Design review of the part built by this model. Coordinates are the model's own, in mm. Face numbers are marked on the shaded views. Give positions to 0.01 mm unless a question says otherwise; leave off trailing zeros. Write each loop counter-clockwise with the first axis right and the second up, starting at its lowest first coordinate (ties: lowest second). Pieces come first, ordered by that corner, then holes. Notation, with made-up numbers: (-6.5, 32) -> (5.5, 32) arc R14 ccw to (5.5, 54) -> close; hole circle Ø5 at (-6, 48). An arc over 180 degrees is marked (long way). Return JSON: item names as keys, results as strings. Group by question number.
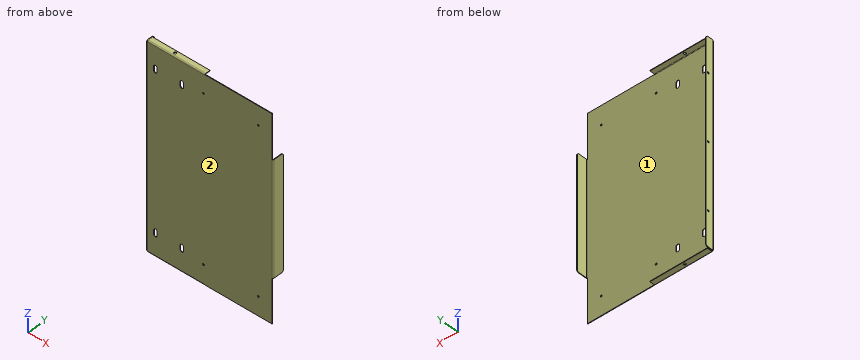
from build123d import *

# Parameters (mm, degrees)
SM_BASE_FLANGE_1_DEPTH   = 381
SKETCH_6_R               = 3.5
CUT_EXTRUDE_1_DEPTH      = 10
SKETCH_7_R               = 3.25
CUT_EXTRUDE_2_DEPTH      = 10
SM_EDGE_FLANGE_2_DEPTH   = 430
OTHER_START              = -2
OTHER_1_DEPTH            = 2
OTHER_START_2            = 477
OTHER_1_2_DEPTH          = 2
SM_START                 = -2
SM_EDGE_FLANGE_4_DEPTH   = 223
SM_EDGE_FLANGE_4_2_DEPTH = 4
SM_START_2               = 220
SM_EDGE_FLANGE_4_3_DEPTH = 1
SM_START_3               = 2
SM_EDGE_FLANGE_4_4_DEPTH = 218
SKETCH_26_R              = 4.5
CUT_EXTRUDE_3_DEPTH      = 905.321292462
SKETCH_28_W              = 762
SKETCH_28_H              = 10
CUT_EXTRUDE_4_DEPTH      = 10
CHAMFER_1_SIZE           = 5


# Read off the part's stored shape, not the designer's step: Затупленный угол1, Ребро-кромка4
# Sheet-metal steps are written as plain solids
with BuildPart() as part:
    # Sketch 1 → Базовая кромка1 (new, symmetric)
    with BuildSketch(Plane.XY):
        with BuildLine():
            Line((0, 40), (0, 2))
            ThreePointArc((0, 2), (0.585786438, 0.585786438), (2, 0))
            Line((2, 0), (475, 0))
            Line((475, 0), (475, -2))
            Line((475, -2), (2, -2))
            ThreePointArc((2, -2), (-0.828427125, -0.828427125), (-2, 2))
            Line((-2, 2), (-2, 40))
            Line((-2, 40), (0, 40))
        make_face()
    extrude(amount=SM_BASE_FLANGE_1_DEPTH, both=True)

    # Эскиз6 → Вырез-Вытянуть1 (cut)
    with BuildSketch(Plane.ZY.offset(2)):
        with Locations(Location((-250, 21, 0), (0, 0, 270))):
            Circle(SKETCH_6_R)
        with Locations(Location((0, 21, 0), (0, 0, 270))):
            Circle(SKETCH_6_R)
        with Locations(Location((250, 21, 0), (0, 0, 270))):
            Circle(SKETCH_6_R)
    extrude(amount=-CUT_EXTRUDE_1_DEPTH, mode=Mode.SUBTRACT)

    # Эскиз7 → Вырез-Вытянуть2 (cut)
    with BuildSketch(Plane.XZ.offset(2)):
        with Locations(Location((215, -310, 0), (0, 0, 270))):
            Circle(SKETCH_7_R)
        with Locations(Location((215, 310, 0), (0, 0, 90))):
            Circle(SKETCH_7_R)
        with Locations(Location((423, -310, 0), (0, 0, 270))):
            Circle(SKETCH_7_R)
        with Locations(Location((423, 310, 0), (0, 0, 90))):
            Circle(SKETCH_7_R)
        with BuildLine():
            Line((26.5, -304), (26.5, -289))
            ThreePointArc((26.5, -289), (33, -282.5), (39.5, -289))
            Line((39.5, -289), (39.5, -304))
            ThreePointArc((39.5, -304), (33, -310.5), (26.5, -304))
        make_face()
        with BuildLine():
            Line((139.5, -289), (139.5, -304))
            ThreePointArc((139.5, -304), (133, -310.5), (126.5, -304))
            Line((126.5, -304), (126.5, -289))
            ThreePointArc((126.5, -289), (133, -282.5), (139.5, -289))
        make_face()
        with BuildLine():
            Line((26.5, 304), (26.5, 289))
            ThreePointArc((26.5, 289), (33, 282.5), (39.5, 289))
            Line((39.5, 289), (39.5, 304))
            ThreePointArc((39.5, 304), (33, 310.5), (26.5, 304))
        make_face()
        with BuildLine():
            Line((139.5, 289), (139.5, 304))
            ThreePointArc((139.5, 304), (133, 310.5), (126.5, 304))
            Line((126.5, 304), (126.5, 289))
            ThreePointArc((126.5, 289), (133, 282.5), (139.5, 289))
        make_face()
    extrude(amount=-CUT_EXTRUDE_2_DEPTH, mode=Mode.SUBTRACT)

    # Ребро-кромка2 section (across the edge) → Ребро-кромка2 (add)
    with BuildSketch(Plane(origin=(477, 0, 215), x_dir=(-1, 0, 0), z_dir=(0, 0, -1))):
        with BuildLine():
            Line((-2, 2), (-2, 40))
            Line((-2, 40), (0, 40))
            Line((0, 40), (0, 2))
            ThreePointArc((0, 2), (0.585786438, 0.585786438), (2, 0))
            Line((2, 0), (2, -2))
            ThreePointArc((2, -2), (-0.828427125, -0.828427125), (-2, 2))
        make_face()
    extrude(amount=SM_EDGE_FLANGE_2_DEPTH)

    # Other 1 outline → Other 1 (cut)
    with BuildSketch(Plane.YZ.offset(OTHER_START)):
        Polygon((40, -381), (40, -376), (35, -381), align=None)
        Polygon((35, 381), (40, 376), (40, 381), align=None)
    extrude(amount=OTHER_1_DEPTH, mode=Mode.SUBTRACT)

    # Other 1 2 outline → Other 1 2 (cut)
    with BuildSketch(Plane.YZ.offset(OTHER_START_2)):
        Polygon((35, 215), (40, 210), (40, 215), align=None)
        Polygon((35, -215), (40, -215), (40, -210), align=None)
    extrude(amount=OTHER_1_2_DEPTH, mode=Mode.SUBTRACT)

    # Ребро-кромка4 outline → Ребро-кромка4 (cut)
    with BuildSketch(Plane.YZ.offset(SM_START)):
        with BuildLine():
            ThreePointArc((0, -379), (0.585786438, -380.414213562), (2, -381))
            Line((2, -381), (2, -379))
            Line((2, -379), (0, -379))
        make_face()
        with BuildLine():
            ThreePointArc((-1.464101616, -381), (-1.863703305, -380.03527618), (-2, -379))
            Line((-2, -379), (-2, -381))
            Line((-2, -381), (-1.464101616, -381))
        make_face()
        with BuildLine():
            ThreePointArc((2, 381), (0.585786438, 380.414213562), (0, 379))
            Line((0, 379), (2, 379))
            Line((2, 379), (2, 381))
        make_face()
        with BuildLine():
            Line((-2, 381), (-2, 379))
            ThreePointArc((-2, 379), (-1.863703305, 380.03527618), (-1.464101616, 381))
            Line((-1.464101616, 381), (-2, 381))
        make_face()
    extrude(amount=SM_EDGE_FLANGE_4_DEPTH, mode=Mode.SUBTRACT)

    # Sm Edge Flange 4 2 outline → Sm Edge Flange 4 2 (cut)
    with BuildSketch(Plane.YZ.offset(SM_START)):
        with BuildLine():
            ThreePointArc((2, -381), (0.585786438, -380.414213562), (0, -379))
            Line((0, -379), (-2, -379))
            ThreePointArc((-2, -379), (-1.863703305, -380.03527618), (-1.464101616, -381))
            Line((-1.464101616, -381), (2, -381))
        make_face()
        with BuildLine():
            Line((2, 381), (-1.464101616, 381))
            ThreePointArc((-1.464101616, 381), (-1.863703305, 380.03527618), (-2, 379))
            Line((-2, 379), (0, 379))
            ThreePointArc((0, 379), (0.585786438, 380.414213562), (2, 381))
        make_face()
    extrude(amount=SM_EDGE_FLANGE_4_2_DEPTH, mode=Mode.SUBTRACT)

    # Sm Edge Flange 4 3 outline → Sm Edge Flange 4 3 (cut)
    with BuildSketch(Plane.YZ.offset(SM_START_2)):
        with BuildLine():
            Line((0, -381), (0, -378))
            Line((0, -378), (-2, -378))
            Line((-2, -378), (-2, -379))
            ThreePointArc((-2, -379), (-1.863703305, -380.03527618), (-1.464101616, -381))
            Line((-1.464101616, -381), (0, -381))
        make_face()
        with BuildLine():
            Line((-2, 378), (0, 378))
            Line((0, 378), (0, 381))
            Line((0, 381), (-1.464101616, 381))
            ThreePointArc((-1.464101616, 381), (-1.863703305, 380.03527618), (-2, 379))
            Line((-2, 379), (-2, 378))
        make_face()
    extrude(amount=SM_EDGE_FLANGE_4_3_DEPTH, mode=Mode.SUBTRACT)

    # Sm Edge Flange 4 4 outline → Sm Edge Flange 4 4 (add)
    with BuildSketch(Plane.YZ.offset(SM_START_3)):
        with BuildLine():
            Line((0, -379), (0, -381))
            Line((0, -381), (-1.464101616, -381))
            ThreePointArc((-1.464101616, -381), (0, -382.464101615), (2, -383))
            Line((2, -383), (20, -383))
            Line((20, -383), (20, -381))
            Line((20, -381), (2, -381))
            ThreePointArc((2, -381), (0.585786438, -380.414213562), (0, -379))
        make_face()
        with BuildLine():
            Line((0, 381), (0, 379))
            ThreePointArc((0, 379), (0.585786438, 380.414213562), (2, 381))
            Line((2, 381), (20, 381))
            Line((20, 381), (20, 383))
            Line((20, 383), (2, 383))
            ThreePointArc((2, 383), (0, 382.464101615), (-1.464101616, 381))
            Line((-1.464101616, 381), (0, 381))
        make_face()
    extrude(amount=SM_EDGE_FLANGE_4_4_DEPTH)

    # Эскиз26 → Вырез-Вытянуть3 (cut, through all)
    with BuildSketch(Plane(origin=(0, 0, -383), x_dir=(-1, 0, 0), z_dir=(0, 0, -1))):
        with Locations(Location((-96, 11, 0), (0, 0, 90))):
            Circle(SKETCH_26_R)
    extrude(amount=-CUT_EXTRUDE_3_DEPTH, mode=Mode.SUBTRACT)

    # Эскиз28 → Вырез-Вытянуть4 (cut)
    with BuildSketch(Plane.ZY.offset(2)):
        with Locations((0, 35)):
            Rectangle(SKETCH_28_W, SKETCH_28_H)
    extrude(amount=-CUT_EXTRUDE_4_DEPTH, mode=Mode.SUBTRACT)

    # Фаска1
    chamfer_1_edges = [part.edges().sort_by_distance(p)[0] for p in [
        (-1, 30, 381),
        (-1, 30, -381),
    ]]
    chamfer(chamfer_1_edges, length=CHAMFER_1_SIZE)


solid = part.part
Q1. Take a section at C-C, the plane x = 448. Give the boundary of the cut face in (y, z).
Q2. For L1, parallel to Z at x = -0.95, y = 21; L2, parallel to Z at x = 204, y = 10; L3, parallel to X at y = -1, z = 310, list the stretches that pass through material, from the lowest coordinate up. Write a range as from..to.
Q3. Take a section at B-B, the plane z = -94. Give the boundary of the cut face in (x, y), plus the area to 3 significant figures.
Q4. Take a section at A-A, the plane x = 115. Give the boundary of the cut face in (y, z), plus the area to 3 significant figures.
Q5. Mouldability with a two-part tool opening along X and no side actions: class the marked faces 1 and 2 as +X half, -X half, draft (parallel to the pull), parting line (faces both ways), or undercut.
Q6. Insertion check: pin 1 (0.6 mm diameter, centred on x = -1, y = 11, fed in from -Z); pin 2 (2 mm diameter, centred on x = -0.5, z = 178.5, fed in from +Y); pin 3 (0.6 mm diameter, centred on y = -1.5, z = 379.5, fed in from -X). Each pin has a flat end and moves straight along its axis. Give the tip position at first contact, or say it passes through.
Final values:
{
 "1": {"outline": "(-2, -381) -> (0, -381) -> (0, 381) -> (-2, 381) -> close"},
 "2": {"L1": "z = -381..-253.5, -246.5..-3.5, 3.5..246.5, 253.5..381", "L2": "z = -383..-381, 381..383", "L3": "x = -0.65..30.5, 35.5..130.5, 135.5..211.75, 218.25..419.75, 426.25..475"},
 "3": {"outline": "(-2, 2) arc R4 ccw to (2, -2) -> (475, -2) arc R4 ccw to (479, 2) -> (479, 40) -> (477, 40) -> (477, 2) arc R2 cw to (475, 0) -> (2, 0) arc R2 cw to (0, 2) -> (0, 30) -> (-2, 30) -> close", "area": "1,100 mm²"},
 "4": {"outline": "(-2, -379) arc R4 ccw to (2, -383) -> (20, -383) -> (20, -381) -> (2, -381) arc R2 cw to (0, -379) -> (0, 379) arc R2 cw to (2, 381) -> (20, 381) -> (20, 383) -> (2, 383) arc R4 ccw to (-2, 379) -> close", "area": "1,610 mm²"},
 "5": {"face 1": "undercut", "face 2": "draft"},
 "6": {"pin 1": "stops at z = -381", "pin 2": "stops at y = 30", "pin 3": "stops at x = 2"}
}
